```python
from build123d import *

# Parameters (mm, degrees)
SKETCH1_W      = 45
SKETCH1_H      = 43.5
EXTRUDE1_DEPTH = 3.175


with BuildPart() as part:
    # Sketch1 → Extrude1 (new body)
    with BuildSketch(Plane(origin=(0, 0, 0), x_dir=(1, 0, 0), z_dir=(0, 1, 0))):
        Polygon((37.227457893, -45.375264395), (37.227457893, -35.375264395), (30.877457893, -35.375264395), (30.877457893, -15.075264395), (22.037457893, -15.075264395), (22.037457893, -16.325264395), (19.787457893, -16.325264395), (19.787457893, -15.075264395), (16.127457893, -15.075264395), (16.127457893, -12.175264395), (19.787457893, -12.175264395), (19.787457893, -10.925264395), (22.037457893, -10.925264395), (22.037457893, -12.175264395), (30.877457893, -12.175264395), (30.877457893, 8.124735605), (36.682921964, 8.124735605), (36.682921964, 18.124735605), (-64.917078036, 18.124735605), (-64.917078036, 8.124735605), (-58.567078036, 8.124735605), (-58.567078036, -12.175264395), (-49.727078036, -12.175264395), (-49.727078036, -10.925264395), (-47.477078036, -10.925264395), (-47.477078036, -12.175264395), (-43.817078036, -12.175264395), (-43.817078036, -15.075264395), (-47.477078036, -15.075264395), (-47.477078036, -16.325264395), (-49.727078036, -16.325264395), (-49.727078036, -15.075264395), (-58.567078036, -15.075264395), (-58.567078036, -35.375264395), (-64.917078036, -35.375264395), (-64.917078036, -45.375264395), align=None)
        with Locations((-13.572542107, -13.625264395)):
            Rectangle(SKETCH1_W, SKETCH1_H, mode=Mode.SUBTRACT)
    extrude(amount=EXTRUDE1_DEPTH)


solid = part.part
```
Model file for the job. Use its own axes, mm. A direction names the side the tool comes from. Coordinates: 2 decimals unless noted, no trailing zeros. Loops run counter-clockwise (first coordinate to the right, second up) from the corner with the lowest first, then second, coordinate; pieces in that order, holes last. Notation, with made-up numbers: M 65.25,23 L 71.25,23 A33 ccw 71.25,54 Z; hole C -7,-29 d10. An arc over 180 degrees is marked long. Use CSV: the item, a comma, the result in double quotes. Start each with the question number.
1. Band-saw the part on B-B, the plane x = 29. List the corners of the cut face in (y, z) (3 decimals).
2. Band-saw the part on A-A, the plane z = -7. List the corners of the cut face in (x, y) (3 decimals), then the cut area to 3 significant figures.
3. Two-plate mould, pull along X, no slides. Class faces 1 (the flat face through (-49, 2, 10.925)), 2 (the flat face through (36.683, 2, -13)), 3 (the flat face through (-13, 2, -18.125)): pulls with the +X half, pulls with the -X half, needs draft (parallel to the pull), parting line crosses it, or undercut.
4. Probe probe 1 along X at (y, z) = (2.75, 16); probe 2 along X at (y, z) = (1.65, 8); probe 3 along Z at (x, y) = (-29, 0.25). List the from-to ranges inside material, lowest first. Write a range as [from, to].
5. Tool access for faces 4 (the flat face through (30.877, 2, 25)), 5 (the flat face through (-62, 2, -8.125)), 6 (the flat face through (-37, 0, 13)), 7 (the flat face through (-14, 2, -8.125)): list every direction of +Z, -Z, +X, -X, +Y, -Y with a clear straight run to the whole face (end or side of a thin tool).
6. Flat gauge pins, fed straight in: pin 1 (1 mm diameter, centred on y = 2, z = 16, fed in from -X); pin 2 (1 mm diameter, centred on y = 1.5, z = 25.5, fed in from +X); pin 3 (0.9 mm diameter, centred on y = 1.5, z = 13.5, fed in from +X). Where does each tip first touch, or does it go through?
Entries:
1,outline,"M 0,-18.125 L 3.175,-18.125 L 3.175,12.175 L 0,12.175 Z; M 0,15.075 L 3.175,15.075 L 3.175,45.375 L 0,45.375 Z"
2,outline,"M -58.567,0 L -36.073,0 L -36.073,3.175 L -58.567,3.175 Z; M 8.927,0 L 30.877,0 L 30.877,3.175 L 8.927,3.175 Z"
2,area,"141 mm2"
3,face 1,"undercut"
3,face 2,"pulls with the +X half"
3,face 3,"needs draft"
4,probe 1,"x = [-58.57, -49.73], [-47.48, -36.07], [8.93, 19.79], [22.04, 30.88]"
4,probe 2,"x = [-58.57, -36.07], [8.93, 30.88]"
4,probe 3,"z = [-18.12, -8.12], [35.38, 45.38]"
5,face 4,"+X, +Y, -Y"
5,face 5,"-X, +Y, -Y"
5,face 6,"+Z, -Z, +X, -X, -Y"
5,face 7,"+Y, -Y"
6,pin 1,"stops at x = -58.57"
6,pin 2,"stops at x = 30.88"
6,pin 3,"stops at x = 16.13"
